Source: CAD feature listing. Evaluate the final solid. Frame: model axes, mm. A direction names the side the tool comes from. Give positions to 0.01 mm unless a question says otherwise; leave off trailing zeros. Loops run counter-clockwise (first coordinate to the right, second up) from the corner with the lowest first, then second, coordinate; pieces in that order, holes last.
```python
from build123d import *

# Parameters (mm, degrees)
SKETCH_1_W          = 74
SKETCH_1_H          = 74
EXTRUDE_1_DEPTH     = 31
SKETCH_2_OUTSIDE_W  = 97.83
SKETCH_2_OUTSIDE_H  = 54.83
CUT_EXTRUDE_1_DEPTH = 89.351570444
SKETCH_3_W          = 31.549660128
SKETCH_3_H          = 15.349381196
EXTRUDE_2_DEPTH     = 3
CUT_EXTRUDE_2_DEPTH = 28
SKETCH_6_R          = 2.7
CUT_EXTRUDE_4_DEPTH = 28


with BuildPart() as part:
    # 草图1 → 凸台-拉伸1 (new body)
    with BuildSketch(Plane(origin=(0, 0, 0), x_dir=(1, 0, 0), z_dir=(0, 1, 0))):
        Rectangle(SKETCH_1_W, SKETCH_1_H)
    extrude(amount=EXTRUDE_1_DEPTH)

    # 草图2 outside → 切除-拉伸1 (cut, through all)
    with BuildSketch(Plane.ZY.offset(37)):
        with Locations((0, 15.5)):
            Rectangle(SKETCH_2_OUTSIDE_W, SKETCH_2_OUTSIDE_H)
        Polygon((30, 31), (-30, 31), (-37, 0), (37, 0), align=None, mode=Mode.SUBTRACT)
    extrude(amount=-CUT_EXTRUDE_1_DEPTH, mode=Mode.SUBTRACT)

    # 草图3 → 凸台-拉伸2 (add)
    with BuildSketch(Plane.ZY.offset(37)):
        with Locations((0, 7.674690598)):
            Rectangle(SKETCH_3_W, SKETCH_3_H)
    extrude(amount=EXTRUDE_2_DEPTH)

    # 草图4 → 切除-拉伸2 (cut)
    with BuildSketch(Plane(origin=(0, 31, 0), x_dir=(1, 0, 0), z_dir=(0, 1, 0))):
        Polygon((8.519431151, 37), (-8.519431151, 37), (0, 33.5), align=None)
        Polygon((-8.519431151, 37), (-8.519431151, 30), (0, 33.5), align=None)
        Polygon((0, 33.5), (8.519431151, 30), (8.519431151, 37), align=None)
        Polygon((0, 33.5), (-8.519431151, 30), (8.519431151, 30), align=None)
        Polygon((-8.519431151, -30), (-8.519431151, -37), (0, -33.5), align=None)
        Polygon((0, -33.5), (-8.519431151, -37), (8.519431151, -37), align=None)
        Polygon((0, -33.5), (8.519431151, -37), (8.519431151, -30), align=None)
        Polygon((8.519431151, -30), (-8.519431151, -30), (0, -33.5), align=None)
    extrude(amount=-CUT_EXTRUDE_2_DEPTH, mode=Mode.SUBTRACT)

    # 草图6 → 切除-拉伸4 (cut)
    with BuildSketch(Plane(origin=(0, 3, 0), x_dir=(1, 0, 0), z_dir=(0, 1, 0))):
        with Locations(Location((0, -32.8, 0), (0, 0, 270))):
            Circle(SKETCH_6_R)
        with Locations(Location((0, 32.8, 0), (0, 0, 270))):
            Circle(SKETCH_6_R)
    extrude(amount=-CUT_EXTRUDE_4_DEPTH, mode=Mode.SUBTRACT)


solid = part.part
```
(1) First-contact query: pin 1 (1 mm diameter, centred on y = 13, z = -21, fed in from -X); pin 2 (0.9 mm diameter, centred on x = -38, z = 1.5, fed in from +Y); pin 3 (8.5 mm diameter, centred on x = -0.5, y = 14.5, fed in from -Z); pin 4 (3 mm diameter, centred on y = 23.5, z = 33.5, fed in from -X). Flat tips, straight axial feed; report the tip coordinate or a pass-through.
A:
pin 1: stops at x = -37
pin 2: stops at y = 15.35
pin 3: stops at z = -30
pin 4: passes through
(2) Reachability of faces 5 (the flat face through (-38, 8, -15.775)), 6 (the flat face through (-38, 8, 15.775)), 7 (the flat face through (8.519, 11, -32)) from +Z, -Z, +X, -X, +Y, -Y: full face, straight path, thin tool, end or side. Return the list, or none.
A:
face 5: -Z, -X, +Y, -Y
face 6: +Z, -X, +Y, -Y
face 7: -Z, +Y
(3) Section B-B, the plane z = -32.8. Return the cut outline in (x, y), then the cut area to 3 significant figures.
A:
outline: (-37, 0) - (-2.7, 0) - (-2.7, 3) - (-8.52, 3) - (-8.52, 18.6) - (-37, 18.6) - close; (2.7, 0) - (37, 0) - (37, 18.6) - (8.52, 18.6) - (8.52, 3) - (2.7, 3) - close
area: 1,090 mm2
(4) Section C-C, the plane z = 10. Return the cut outline in (x, y), then the cut area to 3 significant figures.
A:
outline: (-40, 0) - (37, 0) - (37, 31) - (-37, 31) - (-37, 15.35) - (-40, 15.35) - close
area: 2,340 mm2
(5) Mould query, pull axis Z, two halves, no side actions, for faces 1 (the cylindrical face through (0.1, 1.5, 30.1)), 2 (the flat face through (0, 17, -30)), 3 (the flat face through (0, 3, 36)), 4 (the cylindrical face through (0.1, 1.5, -35.5)). Classes: pulls with the +Z half, pulls with the -Z half, needs draft (parallel to the pull), parting line crosses it, or undercut.
A:
face 1: undercut
face 2: pulls with the -Z half
face 3: needs draft
face 4: undercut
(6) Section A-A, the plane x = 0. Return the cut outline in (y, z), then the cut area to 3 significant figures.
A:
outline: (0, -37) - (3, -36.32) - (3, -35.5) - (0, -35.5) - close; (0, -30.1) - (3, -30.1) - (3, -30) - (31, -30) - (31, 30) - (3, 30) - (3, 30.1) - (0, 30.1) - close; (0, 35.5) - (3, 35.5) - (3, 36.32) - (0, 37) - close
area: 1,870 mm2
(7) Section D-D, the plane y = 27. Return the cut outline in (x, z).
A:
outline: (-37, -30.9) - (-8.52, -30.9) - (-8.52, -30) - (8.52, -30) - (8.52, -30.9) - (37, -30.9) - (37, 30.9) - (8.52, 30.9) - (8.52, 30) - (-8.52, 30) - (-8.52, 30.9) - (-37, 30.9) - close
(8) Ray query, line 1 along X through (y, z) = (2.2, 32.8); line 2 along X through (y, z) = (11, 34); line 3 along X through (y, z) = (3.5, 20). Return the intervals inside material, ascending.
A:
line 1: x = -37 to -2.7, 2.7 to 37
line 2: x = -37 to -8.52, 8.52 to 37
line 3: x = -37 to 37
